Source: CAD feature listing. Evaluate the final solid. Frame: model axes, mm. A direction names the side the tool comes from. Round coordinates to 2 decimals unless told otherwise and drop trailing zeros. Write each loop counter-clockwise with the first axis right and the second up, starting at its lowest first coordinate (ties: lowest second). Pieces come first, ordered by that corner, then holes. Notation, with made-up numbers: M 39,49 L 63,49 A32 ccw 63,80 Z; hole C 10,-17 d8. An arc over 180 degrees is marked long. Answer in a Markdown table with one row per item. Add a question column.
Item 1: Cut plane A-A on z = -27. Return loops of the section in (x, y).
Item 2: Material intervals for probe 1 along X at (y, z) = (3, -22); probe 2 along X at (y, z) = (3, -18.5); probe 3 along X at (y, z) = (19, -10), sorted ascending.
Item 3: Cut plane C-C on x = 85. Return loops of the section in (y, z).
Item 4: Set-up query: faces 4 (the face through (121.36, 18.78, 7.78)), 5 (the face through (101.457, 19.317, -23.938)), 6 (the face through (-18.595, 19.219, -8.585)). Return all of +Z, -Z, +X, -X, +Y, -Y with unobstructed straight access to the full face (end or side cutting, diameter ignored); none if empty.
Item 5: Contact query for flat-ended pins moving along their axis: pin 1 (3 mm diameter, centred on y = 6, z = 5.5, fed in from +X); pin 2 (7.5 mm diameter, centred on y = 11, z = -19, fed in from +X); pin 3 (3.5 mm diameter, centred on x = 56.79, y = 19.05, fed in from +Z); pin 4 (4 mm diameter, centred on y = 16.5, z = 6, fed in from -X). Output: stop coordinate, or through.
Item 6: Cut plane D-D on z = -13.5. Give the number of separate pieces and of enclosed holes in the cut face, and give its area (3 significant figures).
Item 7: Cut plane B-B on y = 19.05. Return loops of the section in (x, z), and give its area (3 significant figures).
Item 8: Mould query, pull axis Z, two halves, no side actions, for faces 1 (the face through (57.46, 16.01, -19.32)), 2 (the face through (58, 23, -38.1)), 3 (the face through (101.231, 19.317, -11.238)). Classes: released by +Z, released by -Z, zero draft, split by the parting line, or undercut.
from build123d import *

# Parameters (mm, degrees)
BOSS_EXTRUDE1_DEPTH = 38.1
SKETCH2_R           = 12.065
CUT_EXTRUDE1_DEPTH  = 15.24
SKETCH3_R           = 12.065
CUT_EXTRUDE2_DEPTH  = 15.24
CUT_EXTRUDE3_DEPTH  = 38.1
SKETCH6_R           = 3.1115
CUT_EXTRUDE4_DEPTH  = 46.482


with BuildPart() as part:
    # Sketch1 → Boss-Extrude1 (new body)
    with BuildSketch(Plane(origin=(0, 0, 0), x_dir=(1, 0, 0), z_dir=(0, 1, 0))):
        Polygon((0, 0), (113.579665808, 0), (129.361202535, -15.781536726), (156.301970898, 11.159231637), (129.361202535, 38.1), (-15.781536726, 38.1), (-42.72230509, 11.159231637), (-15.781536726, -15.781536726), align=None)
    extrude(amount=BOSS_EXTRUDE1_DEPTH)

    # Sketch2 → Cut-Extrude1 (cut)
    with BuildSketch(Plane(origin=(-15.781536726, 0, 15.781536726), x_dir=(0.7071067811865477, 0, 0.7071067811865475), z_dir=(-0.7071067811865475, 0, 0.7071067811865477))):
        with Locations((-19.05, 19.05)):
            Circle(SKETCH2_R)
    extrude(amount=-CUT_EXTRUDE1_DEPTH, mode=Mode.SUBTRACT)

    # Sketch3 → Cut-Extrude2 (cut)
    with BuildSketch(Plane(origin=(72.57136963, 0, 72.57136963), x_dir=(0.7071067811865478, 0, -0.7071067811865474), z_dir=(0.7071067811865474, 0, 0.7071067811865478))):
        with Locations((99.362951898, 19.05)):
            Circle(SKETCH3_R)
    extrude(amount=-CUT_EXTRUDE2_DEPTH, mode=Mode.SUBTRACT)

    # Sketch5 → Cut-Extrude3 (cut)
    with BuildSketch(Plane(origin=(0, 38.1, 0), x_dir=(1, 0, 0), z_dir=(0, 1, 0))):
        Polygon((4.151555437, 17.676821295), (20.32, 30.376821295), (20.32, 4.976821295), align=None)
        Polygon((93.259665808, 30.376821295), (93.259665808, 4.976821295), (109.428110371, 17.676821295), align=None)
    extrude(amount=-CUT_EXTRUDE3_DEPTH, mode=Mode.SUBTRACT)

    # Sketch6 → Cut-Extrude4 (cut)
    with BuildSketch(Plane(origin=(0, 0, -38.1), x_dir=(-1, 0, 0), z_dir=(0, 0, -1))):
        with Locations((-56.789832904, 19.05)):
            Circle(SKETCH6_R)
    extrude(amount=-CUT_EXTRUDE4_DEPTH, mode=Mode.SUBTRACT)


solid = part.part
Results below:
| question | item | result |
|---|---|---|
| 1 | outline | M -26.88,0 L 16.02,0 L 16.02,38.1 L -26.88,38.1 Z; M 20.32,0 L 93.26,0 L 93.26,38.1 L 20.32,38.1 Z; M 97.56,0 L 140.46,0 L 140.46,38.1 L 97.56,38.1 Z; hole C 56.79,19.05 d6.22 |
| 2 | probe 1 | -31.88 to 9.66, 20.32 to 93.26, 103.92 to 145.46 |
| 2 | probe 2 | -35.38 to 5.2, 20.32 to 93.26, 108.38 to 148.96 |
| 2 | probe 3 | -41.56 to -34, -20.01 to 13.92, 20.32 to 53.68, 59.9 to 93.26, 99.65 to 133.59, 147.58 to 155.14 |
| 3 | outline | M 0,-38.1 L 38.1,-38.1 L 38.1,0 L 0,0 Z |
| 4 | face 4 | +Z, +Y, -Y |
| 4 | face 5 | +Y, -Y |
| 4 | face 6 | none |
| 5 | pin 1 | x = 141.14 |
| 5 | pin 2 | x = 152.21 |
| 5 | pin 3 | through |
| 5 | pin 4 | x = -18.38 |
| 6 | separate pieces | 3 |
| 6 | enclosed holes | 3 |
| 6 | area | 6,360 mm2 |
| 7 | outline | M -42.72,-11.16 L -15.78,-38.1 L 53.68,-38.1 L 53.68,0 L 0,0 L -15.78,15.78 L -20.72,10.84 L -9.94,0.07 L -27.01,-17 L -37.78,-6.22 Z; M 59.9,-38.1 L 129.36,-38.1 L 156.3,-11.16 L 151.36,-6.22 L 140.59,-17 L 123.52,0.07 L 134.3,10.84 L 129.36,15.78 L 113.58,0 L 59.9,0 Z; hole M 4.15,-17.68 L 20.32,-30.38 L 20.32,-4.98 Z; hole M 93.26,-30.38 L 109.43,-17.68 L 93.26,-4.98 Z |
| 7 | area | 5,850 mm2 |
| 8 | face 1 | zero draft |
| 8 | face 2 | released by -Z |
| 8 | face 3 | undercut |
